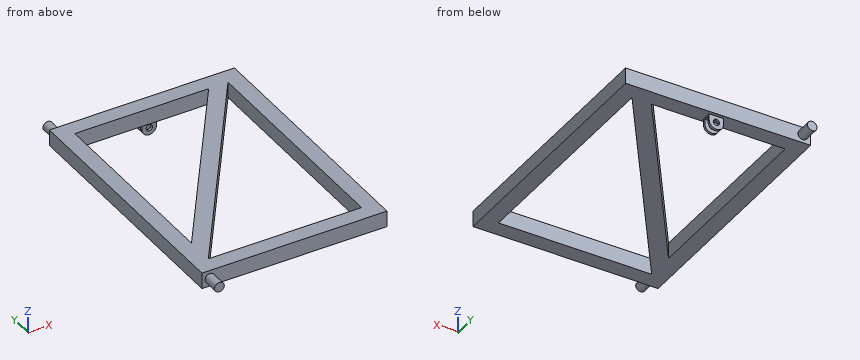
```python
from build123d import *

# Parameters (mm, degrees)
ESQUISSE1_W             = 580
ESQUISSE1_H             = 800
BOSS_EXTRU_1_DEPTH      = 50
ESQUISSE2_R             = 15
BOSS_EXTRU_2_DEPTH      = 50
ESQUISSE3_R             = 15.180649449
BOSS_EXTRU_3_DEPTH      = 50
ESQUISSE4_R             = 10
BOSS_EXTRU_4_DEPTH      = 15
ESQUISSE5_W             = 76.670865877
ESQUISSE5_H             = 44.284034601
ENL_V_MAT_EXTRU_1_DEPTH = 7.5


with BuildPart() as part:
    # Esquisse1 → Boss.-Extru.1 (new body)
    with BuildSketch(Plane.XY):
        with Locations((290, -400)):
            Rectangle(ESQUISSE1_W, ESQUISSE1_H)
        Polygon((50, -50), (469.374013789, -50), (50, -661.587103442), align=None, mode=Mode.SUBTRACT)
        Polygon((530, -50), (530, -750), (50, -750), align=None, mode=Mode.SUBTRACT)
    extrude(amount=BOSS_EXTRU_1_DEPTH)

    # Esquisse2 → Boss.-Extru.2 (add)
    with BuildSketch(Plane(origin=(0, 0, 0), x_dir=(1, 0, 0), z_dir=(0, 1, 0))):
        with Locations(Location((25, -25, 0), (0, 0, 90))):
            Circle(ESQUISSE2_R)
    extrude(amount=BOSS_EXTRU_2_DEPTH)

    # Esquisse3 → Boss.-Extru.3 (add)
    with BuildSketch(Plane.XZ.offset(800)):
        with Locations(Location((25, 25, 0), (0, 0, 90))):
            Circle(ESQUISSE3_R)
    extrude(amount=BOSS_EXTRU_3_DEPTH)

    # Esquisse4 → Boss.-Extru.4 (add, symmetric)
    with BuildSketch(Plane(origin=(0, -25, 0), x_dir=(1, 0, 0), z_dir=(0, 1, 0))):
        with BuildLine():
            Line((311.828309325, -8.678116476), (266.828309325, -8.678116476))
            Line((266.828309325, -8.678116476), (266.828309325, 20))
            ThreePointArc((266.828309325, 20), (289.328309325, 42.5), (311.828309325, 20))
            Line((311.828309325, 20), (311.828309325, -8.678116476))
        make_face()
        with Locations(Location((289.328309325, 20, 0), (0, 0, 270))):
            Circle(ESQUISSE4_R, mode=Mode.SUBTRACT)
    extrude(amount=BOSS_EXTRU_4_DEPTH, both=True)

    # Esquisse5 → Enlèv. mat.-Extru.1 (cut, symmetric)
    with BuildSketch(Plane(origin=(0, -25, 0), x_dir=(1, 0, 0), z_dir=(0, 1, 0))):
        with Locations((288.67808852, 27.082772298)):
            Rectangle(ESQUISSE5_W, ESQUISSE5_H)
    extrude(amount=ENL_V_MAT_EXTRU_1_DEPTH, both=True, mode=Mode.SUBTRACT)


solid = part.part
```
The model under review builds one solid part; all positions refer to its coordinate system, in mm. Round coordinates to 2 decimals unless told otherwise and drop trailing zeros. Loops run counter-clockwise (first coordinate to the right, second up) from the corner with the lowest first, then second, coordinate; pieces in that order, holes last. Notation, with made-up numbers: M -40,19 L 7,19 A18 cw 7,36 Z; hole C 22,64 d5. An arc over 180 degrees is marked long. Put each result on its own line as item: value.
Q1. To check wall thickness, follow L1, parallel to X at y = -241.5, z = 35.5; L2, parallel to X at y = -15.5, z = -20; L3, parallel to Y at x = 353.5, z = 20. State the ranges of each line that lie inside material, in increasing order.
Result set:
L1: x = 0 to 50, 338.06 to 398.69, 530 to 580
L2: x = 266.83 to 279.33, 299.33 to 311.83
L3: y = -800 to -750, -307.4 to -218.98, -50 to 0
Q2. For pin 1 (7.5 mm diameter, centred on x = 294.5, y = -28, fed in from -Z); pin 2 (25 mm diameter, centred on x = 404.5, z = 35, fed in from -Y); pin 3 (13 mm diameter, centred on x = 300.5, z = -26, fed in from -Y); pin 4 (18 mm diameter, centred on x = 289.33, z = -20, fed in from +Y), all flat-tipped, find the tip position at first contact; note any pin that passes through.
Result set:
pin 1: stops at z = -4.94
pin 2: stops at y = -800
pin 3: stops at y = -40
pin 4: passes through
Q3. Consider section A-A, the plane z = 25. Give the boundary of the cut face in (x, y).
Result set:
outline: M 0,-800 L 9.82,-800 L 9.82,-850 L 40.18,-850 L 40.18,-800 L 580,-800 L 580,0 L 40,0 L 40,50 L 10,50 L 10,0 L 0,0 Z; hole M 50,-750 L 530,-750 L 530,-50 Z; hole M 50,-661.59 L 469.37,-50 L 50,-50 Z
Q4. Consider section C-C, the plane x = 90. Give the boundary of the cut face in (y, z).
Result set:
outline: M -800,0 L -750,0 L -750,50 L -800,50 Z; M -691.67,0 L -603.25,0 L -603.25,50 L -691.67,50 Z; M -50,0 L 0,0 L 0,50 L -50,50 Z
Q5. Consider section B-B, the plane y = -699. Give the boundary of the cut face in (x, z).
Result set:
outline: M 0,0 L 84.97,0 L 84.97,50 L 0,50 Z; M 530,0 L 580,0 L 580,50 L 530,50 Z
Q6. Consider section D-D, the plane x = 25. Give the boundary of the cut face in (y, z).
Result set:
outline: M -850,9.82 L -800,9.82 L -800,0 L 0,0 L 0,10 L 50,10 L 50,40 L 0,40 L 0,50 L -800,50 L -800,40.18 L -850,40.18 Z
